```python
from build123d import *

# Parameters (mm, degrees)
F1_DEPTH = 25.4
F2_W     = 19.05
F2_H     = 1.5875
F3_DEPTH = 20.4
F5_DEPTH = 3.175
F6_R     = 1.4
F7_DEPTH = 5
F8_R     = 2.5527
F9_DEPTH = 5


with BuildPart() as f1:
    # F0 (on Top) → F1 (new body)
    with BuildSketch(Plane.XY):
        Polygon((-12.7, -12.025), (-7.7, -12.025), (-7.7, 7.025), (12.7, 7.025), (12.7, 12.025), (-12.7, 12.025), align=None)
    extrude(amount=F1_DEPTH)

    # F2 (on face) → F3 (join)
    with BuildSketch(Plane.YZ.offset(-7.7)):
        with Locations((-2.5, 13.49375)):
            Rectangle(F2_W, F2_H)
        with Locations((-2.5, 11.90625)):
            Rectangle(F2_W, F2_H)
    extrude(amount=F3_DEPTH)

    # F4 (on face) → F5 (cut, through all)
    with BuildSketch(Plane.XY.offset(14.2875)):
        Polygon((-7.7, -12.025), (12.7, -12.025), (12.7, 7.025), (11.35, 7.025), align=None)
    extrude(amount=-F5_DEPTH, mode=Mode.SUBTRACT)

    # F6 (on face) → F7 (cut, through all)
    with BuildSketch(Plane(origin=(0, 12.025, 0), x_dir=(-1, 0, 0), z_dir=(0, 1, 0))):
        with Locations((-6.35, 4.445)):
            Circle(F6_R)
        with Locations((-6.35, 20.955)):
            Circle(F6_R)
        with Locations((3.255, 20.955)):
            Circle(F6_R)
        with Locations((3.255, 4.445)):
            Circle(F6_R)
    extrude(amount=-F7_DEPTH, mode=Mode.SUBTRACT)

    # F8 (on face) → F9 (cut, through all)
    with BuildSketch(Plane(origin=(-12.7, 0, 0), x_dir=(0, -1, 0), z_dir=(-1, 0, 0))):
        with Locations((5.675, 19.05)):
            Circle(F8_R)
        with Locations((5.675, 6.35)):
            Circle(F8_R)
    extrude(amount=-F9_DEPTH, mode=Mode.SUBTRACT)


solid = f1.part
```
Here's how the part is built. I have some questions about the finished solid (model axes, mm). A direction names the side the tool comes from. Give positions to 0.01 mm unless a question says otherwise; leave off trailing zeros. Loops run counter-clockwise (first coordinate to the right, second up) from the corner with the lowest first, then second, coordinate; pieces in that order, holes last. Notation, with made-up numbers: (68.5, -7) -> (81.5, -7) arc R25 cw to (81.5, 16) -> close; hole circle Ø11 at (84.25, 54.25). An arc over 180 degrees is marked (long way). Use one line per item in the form item = value. Start each with the question number.
1) Which directions (+Z, -Z, +X, -X, +Y, -Y) give clear straight access to the entire face, cutting with the end or side of a thin tool? Please do faces 1 (the face through (-12.7, 0, 13)), 2 (the face through (-3, 2, 11.112)), 3 (the face through (2, 7.025, 15)), 4 (the face through (-3, 2, 14.288)).
2) Imagine slicing it at C-C (y = 4). Please give me the cut outline in (x, z) (1 decimal).
3) Thinking about a two-plate mould opening in X: for faces 5 (the face through (12.7, 9, 13)), 6 (the face through (7.46, 9.56, 3.59)), 7 (the face through (-10.24, -5.12, 16.56)), which applies, +X half, -X half, draft (parallel to the pull), parting line (faces both ways), or undercut?
4) Imagine slicing it at D-D (z = 23.75). Please give me the cut outline in (x, y) (3 decimals), then the cut area to 3 significant figures.
5) Imagine slicing it at A-A (z = 6.35). Please give me the cut outline in (x, y) (3 decimals).
6) Imagine slicing it at B-B (x = 6.25). Please give me the cut outline in (y, z) (1 decimal).
7) For P1, Ø3.5, axis at y = 2, z = 18, coming from the +X side; P2, Ø4, axis at x = 6, z = 12, coming from the -Y side (3 decimals); P3, Ø2, axis at x = 4, z = 13, coming from the -Y side (3 decimals), each with a flat end and sliding along its axis, tell me the tip position at first contact or that it passes through.
8) Please list where these lines run through material, in increasing order: line 1 along Y through (x, z) = (4.25, 8.25) (3 decimals); line 2 along Z through (x, y) = (-2.75, -1); line 3 along X through (y, z) = (-8.75, 3.75).
Check values:
q1.face_1 = +Z, -Z, -X, +Y, -Y
q1.face_2 = -Z, +X, -Y
q1.face_3 = +X, -Y
q1.face_4 = +Z, +X, -Y
q2.outline = (-12.7, 0) -> (-7.7, 0) -> (-7.7, 11.1) -> (8.3, 11.1) -> (8.3, 14.3) -> (-7.7, 14.3) -> (-7.7, 25.4) -> (-12.7, 25.4) -> close
q3.face_5 = +X half
q3.face_6 = undercut
q3.face_7 = draft
q4.outline = (-12.7, -12.025) -> (-7.7, -12.025) -> (-7.7, 7.025) -> (12.7, 7.025) -> (12.7, 12.025) -> (-12.7, 12.025) -> close
q4.area = 222 mm^2
q5.outline = (-12.7, -12.025) -> (-7.7, -12.025) -> (-7.7, -8.228) -> (-12.7, -8.228) -> close; (-12.7, -3.122) -> (-7.7, -3.122) -> (-7.7, 7.025) -> (12.7, 7.025) -> (12.7, 12.025) -> (-12.7, 12.025) -> close
q6.outline = (1.9, 11.1) -> (7, 11.1) -> (7, 5.8) -> (12, 5.8) -> (12, 19.6) -> (7, 19.6) -> (7, 14.3) -> (1.9, 14.3) -> close; (7, 0) -> (12, 0) -> (12, 3) -> (7, 3) -> close; (7, 22.4) -> (12, 22.4) -> (12, 25.4) -> (7, 25.4) -> close
q7.P1 = -7.7
q7.P2 = -0.325
q7.P3 = -1.325
q8.line_1 = 7.025 to 12.025
q8.line_2 = 11.11 to 14.29
q8.line_3 = -12.7 to -7.7
